```python
from build123d import *

# Parameters (mm, degrees)
SKETCH1_R           = 2
BOSS_EXTRUDE1_DEPTH = 2
CHAMFER1_SIZE       = 0.3
CUT_EXTRUDE1_DEPTH  = 1.5
CHAMFER2_SIZE       = 0.2
SKETCH3_R           = 1
BOSS_EXTRUDE2_DEPTH = 10
CHAMFER3_SIZE       = 0.2


with BuildPart() as part:
    # Sketch1 → Boss-Extrude1 (new body)
    with BuildSketch(Plane(origin=(0, 0, 0), x_dir=(1, 0, 0), z_dir=(0, 1, 0))):
        with Locations(Location((0, 0, 0), (0, 0, 270))):  # turned: the seam where the file's is
            Circle(SKETCH1_R)
    extrude(amount=BOSS_EXTRUDE1_DEPTH)

    # Chamfer1
    chamfer1_edges = [part.edges().sort_by_distance(p)[0] for p in [
        (0, 2, -2),
    ]]
    chamfer(chamfer1_edges, length=CHAMFER1_SIZE)

    # Sketch2 → Cut-Extrude1 (cut)
    with BuildSketch(Plane(origin=(0, 2, 0), x_dir=(1, 0, 0), z_dir=(0, 1, 0))):
        Polygon((1.154700538, 0), (0.577350269, 1), (-0.577350269, 1), (-1.154700538, 0), (-0.577350269, -1), (0.577350269, -1), align=None)
    extrude(amount=-CUT_EXTRUDE1_DEPTH, mode=Mode.SUBTRACT)

    # Chamfer2
    chamfer2_edges = [part.edges().sort_by_distance(p)[0] for p in [
        (0.866025404, 2, 0.5),
        (0.866025404, 2, -0.5),
        (0, 2, -1),
        (-0.866025404, 2, -0.5),
        (-0.866025404, 2, 0.5),
        (0, 2, 1),
    ]]
    chamfer(chamfer2_edges, length=CHAMFER2_SIZE)

    # Sketch3 → Boss-Extrude2 (add)
    with BuildSketch(Plane.XZ):
        with Locations(Location((0, 0, 0), (0, 0, 90))):  # turned: the seam where the file's is
            Circle(SKETCH3_R)
    extrude(amount=BOSS_EXTRUDE2_DEPTH)

    # Chamfer3
    chamfer3_edges = [part.edges().sort_by_distance(p)[0] for p in [
        (0, -10, -1),
    ]]
    chamfer(chamfer3_edges, length=CHAMFER3_SIZE)


solid = part.part
```
Can you work these out from the model? Positions are in its coordinate system, mm. A direction names the side the tool comes from. Round coordinates to 2 decimals unless told otherwise and drop trailing zeros. Loops run counter-clockwise (first coordinate to the right, second up) from the corner with the lowest first, then second, coordinate; pieces in that order, holes last. Notation, with made-up numbers: M -21.75,-8 L 37.25,-8 A20 ccw 37.25,5 Z; hole C 40,67 d9. An arc over 180 degrees is marked long. Write item = value, one per line. Start each with the question number.
(1) I need wall thicknesses on line 1 along Y through (x, z) = (0.05, -0.4); line 2 along X through (y, z) = (0.5, 1.05); line 3 along Z through (x, y) = (0.05, -3). Which ranges of each line are inside material? Lowest first, please.
(2) If we mould it in two halves opening along Z, with no side actions, what happens to faces 1 (the face through (-2, 1, 0)), 2 (the face through (0, -10, 0)), 3 (the face through (0.86, 1.16, 0.51))? For each: released by +Z, released by -Z, zero draft, split by the parting line, or undercut.
(3) I'm going to push a flat-ended pin straight in: P1, Ø1, axis at x = -0.5, z = 0, coming from the +Y side. Where does the tip first touch, or does it pass through?
(4) Which directions (+Z, -Z, +X, -X, +Y, -Y) give clear straight access to the entire face, cutting with the end or side of a thin tool? Please do faces 4 (the face through (1, 2, 1)), 5 (the face through (1, -5, 0)), 6 (the face through (0, 0.5, 0)).
(5) Suppose I cut it at A-A on x = 0. Write out the boundary of the cut face in (y, z), plus the area to 3 significant figures.
(6) Suppose I cut it at B-B on y = -0.75. Write out the boundary of the cut face in (x, z), plus the area to 3 significant figures.
Answer block:
q1.line_1 = -10 to 0.5
q1.line_2 = -1.7 to 1.7
q1.line_3 = -1 to 1
q2.face_1 = split by the parting line
q2.face_2 = zero draft
q2.face_3 = undercut
q3.P1 = 0.5
q4.face_4 = +Z, -Z, +X, -X, +Y
q4.face_5 = -Y
q4.face_6 = +Y
q5.outline = M -10,-0.8 L -9.8,-1 L 0,-1 L 0,-2 L 1.7,-2 L 2,-1.7 L 2,-1.2 L 1.8,-1 L 0.5,-1 L 0.5,1 L 1.8,1 L 2,1.2 L 2,1.7 L 1.7,2 L 0,2 L 0,1 L -9.8,1 L -10,0.8 Z
q5.area = 24.8 mm²
q6.outline = C 0,0 d2
q6.area = 3.14 mm²
